The figure shows three views and two pictorial views of one solid part (mm, origin at its lowest corner). Answer the questions. A direction names the side the tool comes from. Coordinates: 2 decimals unless noted, no trailing zeros. Order: outer loops, then holes, each group sorted by start corner. A loop starts at its lowest first (then second) coordinate and runs counter-clockwise, first axis right, second up. Notation, with made-up numbers: M 2.5,38.5 L 27.5,38.5 A12 cw 27.5,56.5 Z; hole C 21.5,82.5 d1. An arc over 180 degrees is marked long. Answer in a Markdown table with one row per item. Add a question column.
Item 1: Flat-ended cylindrical pins translate along their axes: pin 1 Ø1.8 at (x, z) = (1.5, 10.5) entering from +Y; pin 2 Ø8 at (y, z) = (13.5, 4) entering from +X; pin 3 Ø6 at (x, z) = (8, 7.5) entering from +Y. Find the tip coordinate at first contact, or state that the pin passes through.
Item 2: The part is cut by section B-B (y = 3.25). Write down the section's boundary in (x, z).
Item 3: The part is cut by section D-D (y = 12). Write down the section's boundary in (x, z), then the cut area to 3 significant figures.
Item 4: Consider line 1 (Z direction, x = 42, y = 0.95); line 2 (X direction, y = 19, z = 8.25); line 3 (Y direction, x = 31, z = 5). Determine where each line is inside the solid, lowest interval first. Write a range as from..to.
Item 5: The mould has two halves that part along X. Classify the marked faces 1, 2 and 3: released by +X, released by -X, zero draft, split by the parting line, or undercut.
Item 6: The part is cut by section A-A (z = 7.75). Write down the section's boundary in (x, y).
Item 7: Which of the six approach directions +Z, -Z, +X, -X, +Y, -Y give full straight-line access (tool end or side, diameter ignored) to the marked faces 4, 5 and 6?
Item 8: The part is cut by section C-C (x = 42). Write down the section's boundary in (y, z).
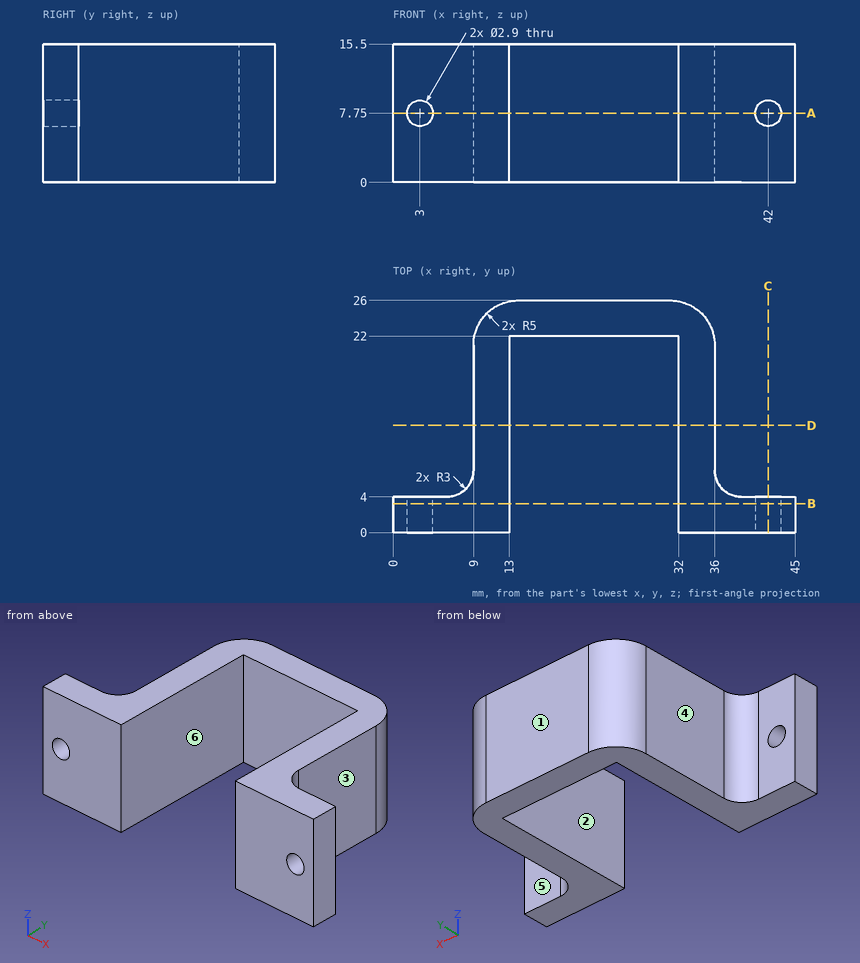
Reply:
| question | item | result |
|---|---|---|
| 1 | pin 1 | stops at y = 4 |
| 1 | pin 2 | stops at x = 36 |
| 1 | pin 3 | stops at y = 25 |
| 2 | outline | M 0,0 L 13,0 L 13,15.5 L 0,15.5 Z; M 32,0 L 45,0 L 45,15.5 L 32,15.5 Z; hole C 3,7.75 d2.9; hole C 42,7.75 d2.9 |
| 3 | outline | M 9,0 L 13,0 L 13,15.5 L 9,15.5 Z; M 32,0 L 36,0 L 36,15.5 L 32,15.5 Z |
| 3 | area | 124 mm2 |
| 4 | line 1 | z = 0..6.3, 9.2..15.5 |
| 4 | line 2 | x = 9..13, 32..36 |
| 4 | line 3 | y = 22..26 |
| 5 | face 1 | zero draft |
| 5 | face 2 | undercut |
| 5 | face 3 | released by +X |
| 6 | outline | M 0,0 L 1.55,0 L 1.55,4 L 0,4 Z; M 4.45,0 L 13,0 L 13,22 L 32,22 L 32,0 L 40.55,0 L 40.55,4 L 39,4 A3 cw 36,7 L 36,21 A5 ccw 31,26 L 14,26 A5 ccw 9,21 L 9,7 A3 cw 6,4 L 4.45,4 Z; M 43.45,0 L 45,0 L 45,4 L 43.45,4 Z |
| 7 | face 4 | +Z, -Z, -X, +Y |
| 7 | face 5 | +Z, -Z, +X, +Y |
| 7 | face 6 | +Z, -Z, -Y |
| 8 | outline | M 0,0 L 4,0 L 4,6.3 L 0,6.3 Z; M 0,9.2 L 4,9.2 L 4,15.5 L 0,15.5 Z |
